The listing builds one solid part. Answer for the finished solid, in the listing's coordinates (mm). Face numbers are marked on the shaded views. A direction names the side the tool comes from. Give positions to 0.01 mm unless a question says otherwise; leave off trailing zeros. Order: outer loops, then holes, each group sorted by start corner. A loop starts at its lowest first (then second) coordinate and runs counter-clockwise, first axis right, second up. Notation, with made-up numbers: (-24.5, -6.5) - (19.5, -6.5) arc R28 ccw to (19.5, 16.5) - close; hole circle Ø2 at (34, -27.5). An arc over 180 degrees is marked (long way). Use CSV: the item, a comma, the result in double quotes.
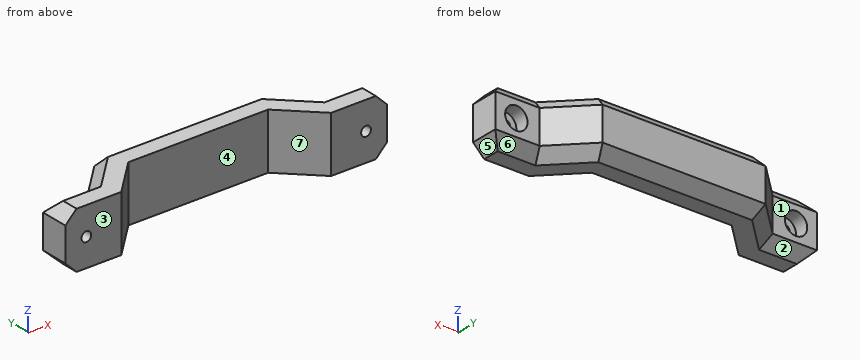
```python
from build123d import *

# Parameters (mm, degrees)
BOSS_EXTRUDE1_DEPTH = 20
CHAMFER1_SIZE       = 4
SKETCH2_R           = 1.75
CUT_EXTRUDE1_DEPTH  = 63.149014473
SKETCH3_R           = 4
CUT_EXTRUDE2_DEPTH  = 5


with BuildPart() as part:
    # Sketch1 → Boss-Extrude1 (new body)
    with BuildSketch(Plane.XY):
        Polygon((-25, 0), (25, 0), (37.5, -12.5), (57.5, -12.5), (57.5, -2.5), (41.642135624, -2.5), (29.142135624, 10), (-29.142135624, 10), (-41.642135624, -2.5), (-57.5, -2.5), (-57.5, -12.5), (-37.5, -12.5), align=None)
    extrude(amount=BOSS_EXTRUDE1_DEPTH)

    # Chamfer1
    chamfer1_edges = [part.edges().sort_by_distance(p)[0] for p in [
        (-57.5, -7.5, 0),
        (-49.571067812, -2.5, 0),
        (-35.392135624, 3.75, 0),
        (0, 10, 0),
        (35.392135624, 3.75, 0),
        (49.571067812, -2.5, 0),
        (57.5, -7.5, 0),
        (57.5, -7.5, 20),
        (49.571067812, -2.5, 20),
        (35.392135624, 3.75, 20),
        (0, 10, 20),
        (-35.392135624, 3.75, 20),
        (-49.571067812, -2.5, 20),
        (-57.5, -7.5, 20),
    ]]
    chamfer(chamfer1_edges, length=CHAMFER1_SIZE)

    # Sketch2 → Cut-Extrude1 (cut, through all)
    with BuildSketch(Plane(origin=(0, -2.5, 0), x_dir=(1, 0, 0), z_dir=(0, 1, 0))):
        with Locations(Location((-50, -10, 0), (0, 0, 180))):
            Circle(SKETCH2_R)
        with Locations(Location((50, -10, 0), (0, 0, 180))):
            Circle(SKETCH2_R)
    extrude(amount=-CUT_EXTRUDE1_DEPTH, mode=Mode.SUBTRACT)

    # Sketch3 → Cut-Extrude2 (cut)
    with BuildSketch(Plane(origin=(0, -2.5, 0), x_dir=(1, 0, 0), z_dir=(0, 1, 0))):
        with Locations(Location((-50, -10, 0), (0, 0, 180))):
            Circle(SKETCH3_R)
        with Locations(Location((50, -10, 0), (0, 0, 180))):
            Circle(SKETCH3_R)
    extrude(amount=-CUT_EXTRUDE2_DEPTH, mode=Mode.SUBTRACT)


solid = part.part
```
Item 1: The mould has two halves that part along X. Classify the marked faces 4, 5, 6 and 7: +X half, -X half, draft (parallel to the pull), parting line (faces both ways), or undercut.
Taken from the geometry:
face 4,"undercut"
face 5,"+X half"
face 6,"draft"
face 7,"undercut"
Item 2: Find the intervals of material crossed by line 1 along Z through (x, y) = (50, -9.15); line 2 along Y through (x, z) = (10.5, 12); line 3 along X through (y, z) = (-3, 17.5), in increasing order.
Taken from the geometry:
line 1,"0 to 8.25, 11.75 to 20"
line 2,"0 to 10"
line 3,"-40.02 to -28, 28 to 40.02"
Item 3: Which of the six approach directions +Z, -Z, +X, -X, +Y, -Y give full straight-line access (tool end or side, diameter ignored) to the marked faces 1, 2 and 3?
Taken from the geometry:
face 1,"+Z, -Z, -X, +Y"
face 2,"-Z, -X, +Y"
face 3,"+Z, -Z, +X, -X, -Y"
Item 4: The part is cut by section C-C (z = 10). Give the vertices of the cut face in (x, y), and give its area (3 significant figures).
Taken from the geometry:
outline,"(-57.5, -12.5) - (-51.75, -12.5) - (-51.75, -7.5) - (-54, -7.5) - (-54, -2.5) - (-57.5, -2.5) - close; (-48.25, -12.5) - (-37.5, -12.5) - (-25, 0) - (25, 0) - (37.5, -12.5) - (48.25, -12.5) - (48.25, -7.5) - (46, -7.5) - (46, -2.5) - (41.64, -2.5) - (29.14, 10) - (-29.14, 10) - (-41.64, -2.5) - (-46, -2.5) - (-46, -7.5) - (-48.25, -7.5) - close; (51.75, -12.5) - (57.5, -12.5) - (57.5, -2.5) - (54, -2.5) - (54, -7.5) - (51.75, -7.5) - close"
area,"1,140 mm^2"
Item 5: The part is cut by section A-A (y = -10.25). Give the vertices of the cut face in (x, z), and give its area (3 significant figures).
Taken from the geometry:
outline,"(-57.5, 4) - (-53.5, 0) - (-35.25, 0) - (-35.25, 20) - (-53.5, 20) - (-57.5, 16) - close; (35.25, 0) - (53.5, 0) - (57.5, 4) - (57.5, 16) - (53.5, 20) - (35.25, 20) - close; hole circle Ø3.5 at (-50, 10); hole circle Ø3.5 at (50, 10)"
area,"839 mm^2"
Item 6: Each of these flat-tipped pins is pushed along its axis until it touches: pin 1 (3.5 mm diameter, centred on x = -51.5, z = 7.5, fed in from +Y); pin 2 (4 mm diameter, centred on y = 4, z = 17, fed in from +X); pin 3 (10 mm diameter, centred on x = -9, z = 7.5, fed in from -Y). Where does it stop, or does it pass through?
Taken from the geometry:
pin 1,"y = -2.5"
pin 2,"x = 36.87"
pin 3,"y = 0"
Item 7: The part is cut by section B-B (x = -50). Give the vertices of the cut face in (y, z), and give its area (4 significant figures).
Taken from the geometry:
outline,"(-12.5, 0) - (-6.5, 0) - (-2.5, 4) - (-2.5, 6) - (-7.5, 6) - (-7.5, 8.25) - (-12.5, 8.25) - close; (-12.5, 11.75) - (-7.5, 11.75) - (-7.5, 14) - (-2.5, 14) - (-2.5, 16) - (-6.5, 20) - (-12.5, 20) - close"
area,"126.5 mm^2"
Item 8: The part is cut by section D-D (x = 17.5). Give the vertices of the cut face in (y, z).
Taken from the geometry:
outline,"(0, 0) - (6, 0) - (10, 4) - (10, 16) - (6, 20) - (0, 20) - close"
